from build123d import *

# Parameters (mm, degrees)
SKETCH2_W           = 220
SKETCH2_H           = 220
BOSS_EXTRUDE1_DEPTH = 6
SKETCH3_R           = 0.5
CUT_EXTRUDE1_DEPTH  = 156.679157243
SKETCH4_R           = 0.5
CUT_EXTRUDE2_DEPTH  = 156.679157243
SKETCH5_W           = 30.4
SKETCH5_H           = 5.6
SKETCH5_W_2         = 5.6
SKETCH5_H_2         = 30.4
CUT_EXTRUDE3_DEPTH  = 156.679157243


with BuildPart() as part:
    # Sketch2 → Boss-Extrude1 (new body)
    with BuildSketch(Plane(origin=(0, 0, 0), x_dir=(1, 0, 0), z_dir=(0, 1, 0))):
        Rectangle(SKETCH2_W, SKETCH2_H)
    extrude(amount=BOSS_EXTRUDE1_DEPTH)

    # Sketch3 → Cut-Extrude1 (cut, through all)
    with BuildSketch(Plane(origin=(0, 6, 0), x_dir=(1, 0, 0), z_dir=(0, 1, 0))):
        with Locations(Location((-77.905, -76, 0), (0, 0, 270))):
            Circle(SKETCH3_R)
        with Locations(Location((-74.095, -76, 0), (0, 0, 270))):
            Circle(SKETCH3_R)
        with Locations(Location((-39.905, -76, 0), (0, 0, 270))):
            Circle(SKETCH3_R)
        with Locations(Location((-36.095, -76, 0), (0, 0, 270))):
            Circle(SKETCH3_R)
        with Locations(Location((-1.905, -76, 0), (0, 0, 270))):
            Circle(SKETCH3_R)
        with Locations(Location((1.905, -76, 0), (0, 0, 270))):
            Circle(SKETCH3_R)
        with Locations(Location((36.095, -76, 0), (0, 0, 270))):
            Circle(SKETCH3_R)
        with Locations(Location((39.905, -76, 0), (0, 0, 270))):
            Circle(SKETCH3_R)
        with Locations(Location((74.095, -76, 0), (0, 0, 270))):
            Circle(SKETCH3_R)
        with Locations(Location((77.905, -76, 0), (0, 0, 270))):
            Circle(SKETCH3_R)
        with Locations(Location((-39.905, -38, 0), (0, 0, 270))):
            Circle(SKETCH3_R)
        with Locations(Location((-36.095, -38, 0), (0, 0, 270))):
            Circle(SKETCH3_R)
        with Locations(Location((-1.905, -38, 0), (0, 0, 270))):
            Circle(SKETCH3_R)
        with Locations(Location((1.905, -38, 0), (0, 0, 270))):
            Circle(SKETCH3_R)
        with Locations(Location((36.095, -38, 0), (0, 0, 270))):
            Circle(SKETCH3_R)
        with Locations(Location((39.905, -38, 0), (0, 0, 270))):
            Circle(SKETCH3_R)
        with Locations(Location((74.095, -38, 0), (0, 0, 270))):
            Circle(SKETCH3_R)
        with Locations(Location((77.905, -38, 0), (0, 0, 270))):
            Circle(SKETCH3_R)
        with Locations(Location((-39.905, 0, 0), (0, 0, 270))):
            Circle(SKETCH3_R)
        with Locations(Location((-36.095, 0, 0), (0, 0, 270))):
            Circle(SKETCH3_R)
        with Locations(Location((-1.905, 0, 0), (0, 0, 270))):
            Circle(SKETCH3_R)
        with Locations(Location((1.905, 0, 0), (0, 0, 270))):
            Circle(SKETCH3_R)
        with Locations(Location((36.095, 0, 0), (0, 0, 270))):
            Circle(SKETCH3_R)
        with Locations(Location((39.905, 0, 0), (0, 0, 270))):
            Circle(SKETCH3_R)
        with Locations(Location((74.095, 0, 0), (0, 0, 270))):
            Circle(SKETCH3_R)
        with Locations(Location((77.905, 0, 0), (0, 0, 270))):
            Circle(SKETCH3_R)
        with Locations(Location((-39.905, 38, 0), (0, 0, 270))):
            Circle(SKETCH3_R)
        with Locations(Location((-36.095, 38, 0), (0, 0, 270))):
            Circle(SKETCH3_R)
        with Locations(Location((-1.905, 38, 0), (0, 0, 270))):
            Circle(SKETCH3_R)
        with Locations(Location((1.905, 38, 0), (0, 0, 270))):
            Circle(SKETCH3_R)
        with Locations(Location((36.095, 38, 0), (0, 0, 270))):
            Circle(SKETCH3_R)
        with Locations(Location((39.905, 38, 0), (0, 0, 270))):
            Circle(SKETCH3_R)
        with Locations(Location((74.095, 38, 0), (0, 0, 270))):
            Circle(SKETCH3_R)
        with Locations(Location((77.905, 38, 0), (0, 0, 270))):
            Circle(SKETCH3_R)
        with Locations(Location((-39.905, 76, 0), (0, 0, 270))):
            Circle(SKETCH3_R)
        with Locations(Location((-36.095, 76, 0), (0, 0, 270))):
            Circle(SKETCH3_R)
        with Locations(Location((-1.905, 76, 0), (0, 0, 270))):
            Circle(SKETCH3_R)
        with Locations(Location((1.905, 76, 0), (0, 0, 270))):
            Circle(SKETCH3_R)
        with Locations(Location((36.095, 76, 0), (0, 0, 270))):
            Circle(SKETCH3_R)
        with Locations(Location((39.905, 76, 0), (0, 0, 270))):
            Circle(SKETCH3_R)
        with Locations(Location((74.095, 76, 0), (0, 0, 270))):
            Circle(SKETCH3_R)
        with Locations(Location((77.905, 76, 0), (0, 0, 270))):
            Circle(SKETCH3_R)
        with Locations(Location((-77.905, -38, 0), (0, 0, 270))):
            Circle(SKETCH3_R)
        with Locations(Location((-74.095, -38, 0), (0, 0, 270))):
            Circle(SKETCH3_R)
        with Locations(Location((-77.905, 0, 0), (0, 0, 270))):
            Circle(SKETCH3_R)
        with Locations(Location((-74.095, 0, 0), (0, 0, 270))):
            Circle(SKETCH3_R)
        with Locations(Location((-77.905, 38, 0), (0, 0, 270))):
            Circle(SKETCH3_R)
        with Locations(Location((-74.095, 38, 0), (0, 0, 270))):
            Circle(SKETCH3_R)
        with Locations(Location((-77.905, 76, 0), (0, 0, 270))):
            Circle(SKETCH3_R)
        with Locations(Location((-74.095, 76, 0), (0, 0, 270))):
            Circle(SKETCH3_R)
    extrude(amount=-CUT_EXTRUDE1_DEPTH, mode=Mode.SUBTRACT)

    # Sketch4 → Cut-Extrude2 (cut, through all)
    with BuildSketch(Plane(origin=(0, 6, 0), x_dir=(1, 0, 0), z_dir=(0, 1, 0))):
        with Locations(Location((84.905, 76, 0), (0, 0, 270))):
            Circle(SKETCH4_R)
        with Locations(Location((88.715, 76, 0), (0, 0, 270))):
            Circle(SKETCH4_R)
        with Locations(Location((92.525, 76, 0), (0, 0, 270))):
            Circle(SKETCH4_R)
        with Locations(Location((96.335, 76, 0), (0, 0, 270))):
            Circle(SKETCH4_R)
        with Locations(Location((100.145, 76, 0), (0, 0, 270))):
            Circle(SKETCH4_R)
        with Locations(Location((-84.905, -76, 0), (0, 0, 270))):
            Circle(SKETCH4_R)
        with Locations(Location((-88.715, -76, 0), (0, 0, 270))):
            Circle(SKETCH4_R)
        with Locations(Location((-92.525, -76, 0), (0, 0, 270))):
            Circle(SKETCH4_R)
        with Locations(Location((-96.335, -76, 0), (0, 0, 270))):
            Circle(SKETCH4_R)
    extrude(amount=-CUT_EXTRUDE2_DEPTH, mode=Mode.SUBTRACT)

    # Sketch5 → Cut-Extrude3 (cut, through all)
    with BuildSketch(Plane(origin=(0, 6, 0), x_dir=(1, 0, 0), z_dir=(0, 1, 0))):
        with Locations((-55, 107.2)):
            Rectangle(SKETCH5_W, SKETCH5_H)
        with Locations((-107.2, -55)):
            Rectangle(SKETCH5_W_2, SKETCH5_H_2)
        with Locations((55, 107.2)):
            Rectangle(SKETCH5_W, SKETCH5_H)
        with Locations((55, -107.2)):
            Rectangle(SKETCH5_W, SKETCH5_H)
        with Locations((-55, -107.2)):
            Rectangle(SKETCH5_W, SKETCH5_H)
        with Locations((-107.2, 55)):
            Rectangle(SKETCH5_W_2, SKETCH5_H_2)
        with Locations((107.2, -55)):
            Rectangle(SKETCH5_W_2, SKETCH5_H_2)
        with Locations((107.2, 55)):
            Rectangle(SKETCH5_W_2, SKETCH5_H_2)
    extrude(amount=-CUT_EXTRUDE3_DEPTH, mode=Mode.SUBTRACT)


solid = part.part
Verification items for the finished model (mm, model axes). A direction names the side the tool comes from. Give positions to 0.01 mm unless a question says otherwise; leave off trailing zeros. Write each loop counter-clockwise with the first axis right and the second up, starting at its lowest first coordinate (ties: lowest second). Pieces come first, ordered by that corner, then holes. Notation, with made-up numbers: M 80.25,88.5 L 112.25,88.5 A6 ccw 112.25,97.5 Z; hole C 10.25,-7 d1. An arc over 180 degrees is marked long. Use CSV: the item, a comma, the result in double quotes.
1) Access from +Z, -Z, +X, -X, +Y, -Y to the whole of each face (thin tool, end or side, straight path). Record for faces 1 (the face through (110, 3, 90)), 2 (the face through (107, 3, -70.2)), 3 (the face through (-39.8, 3, -107)), 4 (the face through (-104.4, 3, -55)), 5 (the face through (-39.8, 3, 107)).
Final values:
face 1,"+Z, -Z, +X, +Y, -Y"
face 2,"+X, +Y, -Y"
face 3,"-Z, +Y, -Y"
face 4,"-X, +Y, -Y"
face 5,"+Z, +Y, -Y"
2) Go/stop test with flat-tipped pins: pin 1 Ø1.8 at (y, z) = (1.5, 62) entering from -X; pin 2 Ø3 at (x, y) = (-59.5, 3.5) entering from -Z; pin 3 Ø3 at (x, y) = (49, 4.5) entering from +Z. Record where each tip stops, or that it passes through.
Final values:
pin 1,"x = -104.4"
pin 2,"z = -104.4"
pin 3,"z = 104.4"
3) Cross-section at A-A (z = 61). Enter the section's corners in (x, y).
Final values:
outline,"M -104.4,0 L 104.4,0 L 104.4,6 L -104.4,6 Z"
4) Cross-section at B-B (y = 3.8). State how many separate pieces and enclosed holes the cut face has, plus the area to 3 significant figures.
Final values:
separate pieces,"1"
enclosed holes,"59"
area,"47,000 mm²"
5) Material ranges on line 1 along Z through (x, y) = (78, 0.45); line 2 along Z through (x, y) = (-40, 1.05); line 3 along Z through (x, y) = (56.5, 2.1), recorded low to high.
Final values:
line 1,"-110 to -76.49, -75.51 to -38.49, -37.51 to -0.49, 0.49 to 37.51, 38.49 to 75.51, 76.49 to 110"
line 2,"-104.4 to -76.49, -75.51 to -38.49, -37.51 to -0.49, 0.49 to 37.51, 38.49 to 75.51, 76.49 to 104.4"
line 3,"-104.4 to 104.4"
6) Release check for a two-part mould opening along Z. For faces 6 (the face through (-90, 3, -110)), 7 (the face through (-104.4, 3, 55)), 8 (the face through (-90, 3, 110)), 9 (the face through (-2, 0, -2)) record: released by +Z, released by -Z, zero draft, split by the parting line, or undercut.
Final values:
face 6,"released by -Z"
face 7,"undercut"
face 8,"released by +Z"
face 9,"zero draft"
